Autodesk Inventor part; units mm, degrees
ref_plane "Work Plane2" through (0, 19.05, 0) normal (0, 1, 0) x (1, 0, 0)
ref_plane "Work Plane1" through (0, 19.05, 0) normal (0, 1, 0) x (1, 0, 0)
ref_plane "YZ Plane" through (0, 0, 0) normal (1, 0, 0) x (0, 1, 0)
sketch "Sketch1" plane through (0, 0, 0) normal (0, 1, 0) x (-1, 0, 0)
  circle A0 centre (0, 0) radius 8.0645
  circle A1 centre (0, -63.5) radius 6.985
  circle A2 centre (0, 63.5) radius 6.985
  line L0 (-39.6048, 88.9) -> (39.6048, 88.9)
  line L1 (39.6048, 88.9) -> (39.6048, -88.9)
  line L2 (39.6048, -88.9) -> (-39.6048, -88.9)
  line L3 (-39.6048, -88.9) -> (-39.6048, 88.9)
  line L4 (-39.6048, 88.9) -> (39.6048, -88.9) construction
  line L5 (39.6048, 88.9) -> (-39.6048, -88.9) construction
  line L6 (10.9754, 63.5) -> (10.9754, 0) construction
  point P0 (0, 0)
  point P1 (0, 0)
  point P2 (0, 63.5)
  dimension "d0" = 16.129
  dimension "d1" = 13.97
  dimension "d2" = 13.97
  dimension "d28" = 177.8
  dimension "d30" = 25.4
  dimension "d31" = 25.4
extrude "Extrusion4" add sketch "Sketch1" along normal blind 19.05
ref_plane "Work Plane2" through (0, 19.05, 0) normal (0, 1, 0) x (1, 0, 0)
sketch "Sketch2" plane through (0, 19.05, 0) normal (0, 1, 0) x (1, 0, 0)
  circle A0 centre (-11.2395, 0) radius 1.25
  circle A1 centre (0, 0) radius 7.94
  circle A2 centre (5.6197, -9.7337) radius 1.25
  circle A3 centre (5.6198, 9.7337) radius 1.25
  dimension "d11" = 2.5
  dimension "d12" = 11.2395
  dimension "d15" = 360
ref_plane "Work Plane1" through (0, 19.05, 0) normal (0, 1, 0) x (1, 0, 0)
extrude "Extrusion5" cut sketch "Sketch2" against normal up to next contours A0 | A2 | A3
sketch "Sketch6" plane through (0, 19.05, 0) normal (0, 1, 0) x (1, 0, 0)
  line L0 (0, -38.1) -> (0, -18.8395)
  line L1 (0, 18.8395) -> (0, 38.1)
  line L2 (39.6048, 88.9) -> (-39.6048, 88.9)
  line L3 (0, 88.9) -> (-39.6048, 88.9)
  line L4 (-39.6048, -88.9) -> (39.6048, -88.9)
  line L5 (-39.6048, 88.9) -> (-39.6048, -88.9)
  line L6 (-39.6048, -88.9) -> (0, -88.9)
  circle A0 centre (0, 0) radius 8.0645
  arc A1 (0, 18.8395) -> (0, -18.8395) centre (0, 0) ccw
  arc A2 (0, -50.8) -> (0, -76.2) centre (0, -63.5) ccw
  line L7 (0, -38.1) -> (0, -50.8)
  line L8 (0, -76.2) -> (0, -88.9)
  arc A3 (0, 76.2) -> (0, 50.8) centre (0, 63.5) ccw
  line L9 (0, 88.9) -> (0, 76.2)
  line L10 (0, 50.8) -> (0, 38.1)
  circle A4 centre (0, 63.5) radius 6.477
  circle A5 centre (0, -63.5) radius 6.477
  circle A6 centre (-11.2395, 0) radius 1.25
  point P0 (0, 0)
  dimension "d41" = 25.4
  dimension "d42" = 25.4
  dimension "d44" = 12.954
  dimension "d45" = 12.954
  dimension "d77" = 6.35
extrude "Extrusion6" cut sketch "Sketch6" against normal blind 19.05 contours L7 A2 L8 L4 L5 L2 L9 A3 L10 L1 A1 L0
fillet "Fillet5" radius 12.7 4 edges at (0, 9.525, 50.8) (0, 9.525, -50.8) (0, 9.525, -18.8395) (0, 9.525, 18.8395)
sketch "Sketch8" plane through (0, 19.05, -88.9) normal (-1, 0, 0) x (0, 0, 1)
  line L0 (33.355, -16.3528) -> (33.355, -2.5052)
  line L1 (15.575, -2.511) -> (15.575, -16.351)
  line L2 (27.5747, -16.3528) -> (27.5747, -2.5052)
  line L3 (21.1759, -16.351) -> (21.1759, -2.511)
  line L4 (33.355, -16.3528) -> (27.5747, -16.3528)
  line L5 (33.355, -2.5052) -> (27.5747, -2.5052)
  line L6 (15.575, -16.351) -> (21.1759, -16.351)
  line L7 (21.1759, -2.511) -> (15.575, -2.511)
  point P0 (88.9, -19.05)
extrude "Extrusion7" cut sketch "Sketch8" along normal up to next
mirror "Mirror1" about plane through (0, 0, 0) normal (0, 0, 1) of "Extrusion7"
fillet "Fillet6" radius 12.7 2 edges at (0, 9.525, 88.9) (0, 9.525, -88.9)
sketch "Sketch12" plane through (0, 19.05, 0) normal (0, 1, 0) x (1, 0, 0)
  line L0 (39.6048, -88.9) -> (39.6048, 88.9)
  line L1 (39.6048, -82.55) -> (19.685, -82.55)
  line L2 (19.685, -82.55) -> (19.685, 82.55)
  line L3 (19.685, 82.55) -> (39.6048, 82.55)
  line L4 (39.6048, 82.55) -> (39.6048, -82.55)
  line L5 (39.6048, 88.9) -> (12.7, 88.9)
  line L6 (12.7, -88.9) -> (39.6048, -88.9)
  circle A0 centre (0, -63.5) radius 6.985
  point P0 (0, 0)
  dimension "d72" = 6.35
  dimension "d73" = 6.35
  dimension "d74" = 12.7
extrude "Extrusion10" cut sketch "Sketch12" against normal up to next contours L1 L2 L3 L0
sketch "Sketch13" plane through (39.6048, 0, 88.9) normal (1, 0, 0) x (0, 0, -1)
  line L0 (0, 0) -> (0, 19.05)
  line L1 (171.45, 0) -> (6.35, 0)
  line L2 (0, 19.05) -> (6.35, 19.05)
  line L3 (6.35, 19.05) -> (6.35, 0)
  line L4 (6.35, 0) -> (0, 0)
  line L5 (0, 0) -> (0, 19.05)
  line L6 (171.45, 19.05) -> (171.45, 0)
  line L7 (177.8, 19.05) -> (177.8, 0)
  line L8 (171.45, 19.05) -> (177.8, 19.05)
  line L9 (177.8, 19.05) -> (177.8, 0)
  line L10 (177.8, 0) -> (171.45, 0)
  line L11 (171.45, 0) -> (171.45, 19.05)
  point P0 (88.9, 0)
extrude "Extrusion11" add sketch "Sketch13" along normal blind 50.8
properties part number "AlteredPlatform"
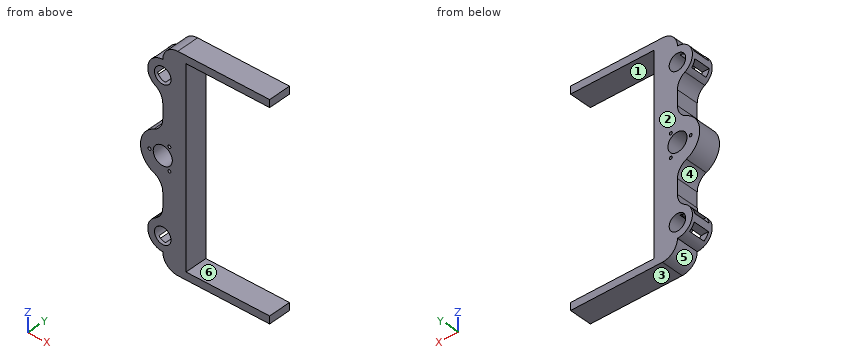
For this review, take the finished solid that the model builds, in its own axes (mm). Face numbers are marked on the shaded views. A direction names the side the tool comes from. Coordinates: 2 decimals unless noted, no trailing zeros. Write each loop counter-clockwise with the first axis right and the second up, starting at its lowest first coordinate (ties: lowest second). Pieces come first, ordered by that corner, then holes. Notation, with made-up numbers: (-9.75, 49) -> (41.25, 49) arc R28 ccw to (41.25, 88) -> close; hole circle Ø5 at (7, 57.5). An arc over 180 degrees is marked (long way). Put each result on its own line as item: value.
Q1. Wall thickness on L1, parallel to Z at x = -1.5, y = 9.5 (3 decimals); L2, parallel to Z at x = -5, y = 1; L3, parallel to Z at x = 38, y = 9.25: over which ranges is each line inside the solid? List them lowest first.
From the geometry:
L1: z = -76.111 to -73.325, -55.545 to -47.49, -22.882 to -7.924, 7.924 to 22.882, 47.49 to 55.545, 73.325 to 76.111
L2: z = -75.17 to -68.38, -58.62 to -51.6, -18.77 to -6.33, 6.33 to 18.77, 51.6 to 58.62, 68.38 to 75.17
L3: z = -88.9 to -82.55, 82.55 to 88.9
Q2. The part is to be moulded in two halves that separate along Z. For the marked faces 1, 2 and 3, say which applies: +Z half, -Z half, draft (parallel to the pull), parting line (faces both ways), or undercut.
From the geometry:
face 1: undercut
face 2: draft
face 3: -Z half
Q3. Take a section at A-A, the plane z = -63.5. State the section outline as (x, y) points (3 decimals), then the cut area to 3 significant figures.
From the geometry:
outline: (-12.7, 0) -> (-6.985, 0) -> (-6.985, 19.05) -> (-12.7, 19.05) -> close; (6.985, 0) -> (19.685, 0) -> (19.685, 19.05) -> (6.985, 19.05) -> close
area: 351 mm2
Q4. Take a section at D-D, the plane z = -31.5. State the section outline as (x, y) points (3 decimals).
From the geometry:
outline: (0, 0) -> (19.685, 0) -> (19.685, 19.05) -> (0, 19.05) -> close
Q5. Tool access review of the marked faces 4, 5 and 6: name each direction out of +Z, -Z, +X, -X, +Y, -Y from which nothing blocks a thin tool from reaching the whole face with its end or side.
From the geometry:
face 4: -X, +Y, -Y
face 5: -Z, -X, +Y, -Y
face 6: +X, +Y, -Y
Q6. Take a section at C-C, the plane y = 11.75. Count the separate pieces of the cut face and the enclosed holes in it, then the cut area to 3 significant figures.
From the geometry:
separate pieces: 3
enclosed holes: 4
area: 4,750 mm2
Q7. Clearance check with flat-ended pins moving along their axes: pin 1 Ø4.5 at (x, z) = (-5, -69.5) entering from -Y; pin 2 Ø2.5 at (x, y) = (-2, 8) entering from -Z; pin 3 Ø2 at (y, z) = (9, 41.5) entering from -X; pin 4 Ø3 at (x, y) = (-5, 10) entering from -Z. State where each tip first meets the part, or that it passes through.
From the geometry:
pin 1: stops at y = 0
pin 2: stops at z = -76.18
pin 3: stops at x = -0.04
pin 4: stops at z = -75.71
Q8. Take a section at B-B, the plane x = 74.5. State the section outline as (y, z) points.
From the geometry:
outline: (0, -88.9) -> (19.05, -88.9) -> (19.05, -82.55) -> (0, -82.55) -> close; (0, 82.55) -> (19.05, 82.55) -> (19.05, 88.9) -> (0, 88.9) -> close
